```python
from build123d import *

# Parameters (mm, degrees)
F0_R     = 2.5
F0_R_2   = 2.032
F1_DEPTH = 9
F3_DEPTH = 9.001
F4_R     = 1.25
F5_DEPTH = 4.501


with BuildPart() as f1:
    # F0 (on Top) → F1 (new body)
    with BuildSketch(Plane.XY):
        with BuildLine():
            Line((0, 4.5), (-50, 4.5))
            ThreePointArc((-50, 4.5), (-54.5, 0), (-50, -4.5))
            Line((-50, -4.5), (0, -4.5))
            ThreePointArc((0, -4.5), (4.5, 0), (0, 4.5))
        make_face()
        with Locations((-50, 0)):
            Circle(F0_R, mode=Mode.SUBTRACT)
        Circle(F0_R_2, mode=Mode.SUBTRACT)
    extrude(amount=F1_DEPTH)

    # F2 (on face) → F3 (cut, through all)
    with BuildSketch(Plane.XZ.offset(4.5)):
        Polygon((-98.52826, 9), (-94.756936, 2), (-11.5, 2), (-4.5, 9), align=None)
    extrude(amount=-F3_DEPTH, mode=Mode.SUBTRACT)

    # F4 (on Right) → F5 (cut, through all)
    with BuildSketch(Plane.YZ):
        with Locations((0, 4.5)):
            Circle(F4_R)
    extrude(amount=F5_DEPTH, mode=Mode.SUBTRACT)


solid = f1.part
```
Model file for the job. Use its own axes, mm. A direction names the side the tool comes from. Give positions to 0.01 mm unless a question says otherwise; leave off trailing zeros. Order: outer loops, then holes, each group sorted by start corner. A loop starts at its lowest first (then second) coordinate and runs counter-clockwise, first axis right, second up.
1) Saw through at B-B, the plane y = 0. Write the cut outline in (x, z), then the cut area to 3 significant figures.
2) 3-axis set-ups, long thin cutter, end or side, ignore diameter. For faces 4 (the flat face through (-33, 0, 2)), 5 (the flat face through (-2, -1, 9)): which of +Z, -Z, +X, -X, +Y, -Y reach the whole face in a straight line?
3) Saw through at A-A, the plane x = -48. Write the cut outline in (y, z).
4) Pin check, flat tips, straight feed: pin 1 (1.5 mm diameter, centred on x = -13.5, y = 2.5, fed in from +Z); pin 2 (4 mm diameter, centred on y = 0, z = 4.5, fed in from -X); pin 3 (1 mm diameter, centred on y = -2, z = 8, fed in from +X). Stop position of each tip, or through.
5) Saw through at D-D, the plane x = -39. Write the cut outline in (y, z), then the cut area to 3 significant figures.
6) Saw through at C-C, the plane z = 2.5. Write the cut outline in (x, y).
7) Mould opens along Y. For faces 1 (the flat face through (-8, -0.1, 5.5)), 2 (the cylindrical face through (3.033, 1.155, 4.021)), 3 (the cylindrical face through (4.194, -1.632, 4.437)) say: +Y half, -Y half, draft (parallel to the pull), parting line (faces both ways), or undercut.
8) Wall check: probe 1 along Y at (x, z) = (0, 5.25); probe 2 along X at (y, z) = (1.5, 1.25); probe 3 along Z at (x, y) = (-32.5, 1.75). Give the ranges that are in metal, low to high.
Computed:
1. outline: (-54.5, 0) - (-52.5, 0) - (-52.5, 2) - (-54.5, 2) - close; (-47.5, 0) - (-2.03, 0) - (-2.03, 9) - (-4.5, 9) - (-11.5, 2) - (-47.5, 2) - close; (2.03, 0) - (4.5, 0) - (4.5, 3.25) - (2.03, 3.25) - close; (2.03, 5.75) - (4.5, 5.75) - (4.5, 9) - (2.03, 9) - close
1. area: 153 mm2
2. face 4: +Z, -X, +Y, -Y
2. face 5: +Z, +X, -X, +Y, -Y
3. outline: (-4.5, 0) - (-1.5, 0) - (-1.5, 2) - (-4.5, 2) - close; (1.5, 0) - (4.5, 0) - (4.5, 2) - (1.5, 2) - close
4. pin 1: stops at z = 2
4. pin 2: stops at x = -11
4. pin 3: stops at x = 4.24
5. outline: (-4.5, 0) - (4.5, 0) - (4.5, 2) - (-4.5, 2) - close
5. area: 18.0 mm2
6. outline: (-11, -4.5) - (0, -4.5) arc R4.5 ccw to (0, 4.5) - (-11, 4.5) - close; hole circle Ø4.06 at (0, 0)
7. face 1: draft
7. face 2: undercut
7. face 3: parting line
8. probe 1: y = -4.5 to -2.03, 2.03 to 4.5
8. probe 2: x = -54.24 to -52, -48 to -1.37, 1.37 to 4.24
8. probe 3: z = 0 to 2
